from build123d import *

# Parameters (mm, degrees)
SKETCH1_W           = 150
SKETCH1_H           = 20
BOSS_EXTRUDE1_DEPTH = 5
SKETCH3_W           = 150
SKETCH3_H           = 5
BOSS_EXTRUDE2_DEPTH = 15
SKETCH5_R           = 2
CUT_EXTRUDE1_DEPTH  = 6
SKETCH6_R           = 2
CUT_EXTRUDE2_DEPTH  = 6
SKETCH7_W           = 150
SKETCH7_H           = 5
BOSS_EXTRUDE3_DEPTH = 10


with BuildPart() as part:
    # Sketch1 → Boss-Extrude1 (new body)
    with BuildSketch(Plane(origin=(0, 0, 0), x_dir=(1, 0, 0), z_dir=(0, 1, 0))):
        with Locations((75, 10)):
            Rectangle(SKETCH1_W, SKETCH1_H)
    extrude(amount=-BOSS_EXTRUDE1_DEPTH)

    # Sketch3 → Boss-Extrude2 (add)
    with BuildSketch(Plane(origin=(0, 0, 0), x_dir=(1, 0, 0), z_dir=(0, 1, 0))):
        with Locations((75, 17.5)):
            Rectangle(SKETCH3_W, SKETCH3_H)
    extrude(amount=BOSS_EXTRUDE2_DEPTH)

    # Sketch5 → Cut-Extrude1 (cut, through all)
    with BuildSketch(Plane.XY.offset(-15)):
        with Locations((25, 7.5)):
            Circle(SKETCH5_R)
        with Locations((125, 7.5)):
            Circle(SKETCH5_R)
    extrude(amount=-CUT_EXTRUDE1_DEPTH, mode=Mode.SUBTRACT)

    # Sketch6 → Cut-Extrude2 (cut, through all)
    with BuildSketch(Plane(origin=(0, 0, 0), x_dir=(1, 0, 0), z_dir=(0, 1, 0))):
        with Locations((35, 2.1)):
            Circle(SKETCH6_R)
        with Locations((115, 2.1)):
            Circle(SKETCH6_R)
    extrude(amount=-CUT_EXTRUDE2_DEPTH, mode=Mode.SUBTRACT)

    # Sketch7 → Boss-Extrude3 (add)
    with BuildSketch(Plane.XY):
        with Locations((75, -2.5)):
            Rectangle(SKETCH7_W, SKETCH7_H)
    extrude(amount=BOSS_EXTRUDE3_DEPTH)


solid = part.part
Input: part model. Units: mm. Frame: model coordinates. A direction names the side the tool comes from. Round coordinates to 2 decimals unless told otherwise and drop trailing zeros. Order: outer loops, then holes, each group sorted by start corner. A loop starts at its lowest first (then second) coordinate and runs counter-clockwise, first axis right, second up. Notation, with made-up numbers: (61, -5) - (77, -5) arc R17 ccw to (77, 2) - close; hole circle Ø10 at (25.25, 74.25). An arc over 180 degrees is marked (long way). Answer as a JSON object with one key per item and string values. Group by question number.
(1) Cut plane B-B (z = -2.1). Return loops of the section in (x, y).
(2) Cut plane A-A (x = 115). Return loops of the section in (y, z).
(3) Pin query (flat end, axial travel): P1, Ø3, axis at x = 115, z = -2.1, coming from the +Y side; P2, Ø4.5, axis at x = 25, y = 7.5, coming from the +Z side; P3, Ø1.5, axis at x = 16, z = -12.5, coming from the +Y side. Return the tip coordinate at first contact, or that it passes through.
(4) Material intervals for probe 1 along X at (y, z) = (-1.9, -2.1); probe 2 along Z at (x, y) = (35, -1.6); probe 3 along Y at (x, z) = (60.5, -6.75), sorted ascending. Write a range as from..to.
(5) Cut plane C-C (y = 7.5). Return loops of the section in (x, z).
(6) Reachability of faces 1 (the face through (74, -5, -5)), 2 (the face through (74, 0, -3)) from +Z, -Z, +X, -X, +Y, -Y: full face, straight path, thin tool, end or side. Return the list, or none.
(7) Cut plane D-D (x = 131.5). Return loops of the section in (y, z), then the cut area to 3 significant figures.
(8) Draft query along Z for faces 3 (the face through (74, 5, -20)), 4 (the face through (113.002, -2.465, -2.188)), 5 (the face through (36.908, -2.465, -2.701)), 6 (the face through (123.002, 7.588, -17.465)). Return one class per face: released by +Z, released by -Z, zero draft, split by the parting line, or undercut.
Here are the results:
{
 "1": {"outline": "(0, -5) - (33, -5) - (33, 0) - (0, 0) - close; (37, -5) - (113, -5) - (113, 0) - (37, 0) - close; (117, -5) - (150, -5) - (150, 0) - (117, 0) - close"},
 "2": {"outline": "(-5, -20) - (15, -20) - (15, -15) - (0, -15) - (0, -4.1) - (-5, -4.1) - close; (-5, -0.1) - (0, -0.1) - (0, 10) - (-5, 10) - close"},
 "3": {"P1": "passes through", "P2": "stops at z = -15", "P3": "stops at y = 0"},
 "4": {"probe 1": "x = 0..33, 37..113, 117..150", "probe 2": "z = -20..-4.1, -0.1..10", "probe 3": "y = -5..0"},
 "5": {"outline": "(0, -20) - (23, -20) - (23, -15) - (0, -15) - close; (27, -20) - (123, -20) - (123, -15) - (27, -15) - close; (127, -20) - (150, -20) - (150, -15) - (127, -15) - close"},
 "6": {"face 1": "+Z, -Z, +X, -X, -Y", "face 2": "+Z, +X, -X, +Y"},
 "7": {"outline": "(-5, -20) - (15, -20) - (15, -15) - (0, -15) - (0, 10) - (-5, 10) - close", "area": "225 mm^2"},
 "8": {"face 3": "released by -Z", "face 4": "undercut", "face 5": "undercut", "face 6": "zero draft"}
}
